Design review of the part built by this model. Coordinates are the model's own, in mm. Face numbers are marked on the shaded views. A direction names the side the tool comes from. Give positions to 0.01 mm unless a question says otherwise; leave off trailing zeros. Write each loop counter-clockwise with the first axis right and the second up, starting at its lowest first coordinate (ties: lowest second). Pieces come first, ordered by that corner, then holes. Notation, with made-up numbers: M 43,61 L 71,61 A15 cw 71,73 Z; hole C 81.25,68.25 d10. An arc over 180 degrees is marked long. One line per item, written item: value. Start each with the question number.
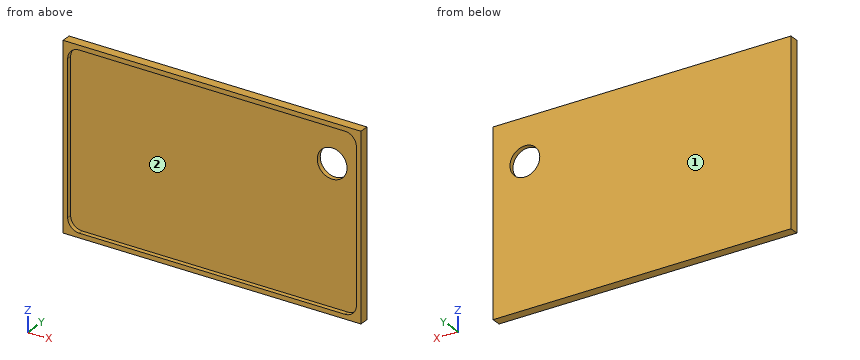
```python
from build123d import *

# Parameters (mm, degrees)
SKETCH1_W           = 65
SKETCH1_H           = 40
BOSS_EXTRUDE1_DEPTH = 45
SHELL1_T            = -1
SKETCH2_R           = 5
CUT_EXTRUDE1_DEPTH  = 8
SKETCH3_R           = 7.5
CUT_EXTRUDE2_DEPTH  = 8
FILLET1_R           = 2
FILLET2_R           = 2.5
SKETCH5_W           = 66.843722153
SKETCH5_H           = 46.578661822
CUT_EXTRUDE3_DEPTH  = 250
SKETCH7_W           = 65
SKETCH7_H           = 40
BOSS_EXTRUDE3_DEPTH = 1
SKETCH8_R           = 3.25
CUT_EXTRUDE4_DEPTH  = 7


with BuildPart() as part:
    # Sketch1 → Boss-Extrude1 (new body)
    with BuildSketch(Plane(origin=(0, 0, 0), x_dir=(1, 0, 0), z_dir=(0, 1, 0))):
        Rectangle(SKETCH1_W, SKETCH1_H)
    extrude(amount=BOSS_EXTRUDE1_DEPTH)

    # Shell1
    shell1_openings = [part.faces().sort_by_distance(p)[0] for p in [
        (0, 45, 0),
    ]]
    offset(amount=SHELL1_T, openings=shell1_openings, kind=Kind.INTERSECTION)

    # Sketch2 → Cut-Extrude1 (cut)
    with BuildSketch(Plane(origin=(32.5, 0, 0), x_dir=(0, 0, -1), z_dir=(1, 0, 0))):
        with Locations((0, 26)):
            Circle(SKETCH2_R)
    extrude(amount=-CUT_EXTRUDE1_DEPTH, mode=Mode.SUBTRACT)

    # Sketch3 → Cut-Extrude2 (cut)
    with BuildSketch(Plane.XZ):
        with Locations(Location((0, 0, 0), (0, 0, 270))):
            Circle(SKETCH3_R)
    extrude(amount=-CUT_EXTRUDE2_DEPTH, mode=Mode.SUBTRACT)

    # Fillet1
    # the kernel refuses this fillet: 2 mm, written as the material it adds along each edge
    with BuildSketch(Plane(origin=(31.5, 1, 19), x_dir=(0, 1, 0), z_dir=(0, 0, -1)), Plane(origin=(-31.5, 1, -19), x_dir=(0, 1, 0), z_dir=(0, 0, 1))) as fillet1_piece_1:
        with BuildLine():
            CenterArc((FILLET1_R, -FILLET1_R), FILLET1_R, 90, 90)
            Line((0, -FILLET1_R), (0, 0))
            Line((0, 0), (FILLET1_R, 0))
        make_face()
    extrude(amount=38)
    with BuildSketch(Plane(origin=(31.5, 1, -19), x_dir=(0, 1, 0), z_dir=(-1, 0, 0)), Plane(origin=(-31.5, 1, 19), x_dir=(0, 1, 0), z_dir=(1, 0, 0))) as fillet1_piece_2:
        with BuildLine():
            CenterArc((FILLET1_R, -FILLET1_R), FILLET1_R, 90, 90)
            Line((0, -FILLET1_R), (0, 0))
            Line((0, 0), (FILLET1_R, 0))
        make_face()
    extrude(amount=63)
    # the kernel refuses this fillet: 2 mm, written as the material it takes off along each edge
    with BuildSketch(Plane(origin=(0, 1, 0), x_dir=(0, 0, -1), z_dir=(-1, 0, 0))) as fillet1_2_piece_1:
        with BuildLine():
            CenterArc((9.232050808, 2), FILLET1_R, 210, 60)
            Line((9.232050808, 0), (7.5, 0))
            Line((7.5, 0), (7.5, 1))
        make_face()
    revolve(axis=Axis((0, 1, 0), (0, -1, 0)), mode=Mode.SUBTRACT)

    # Fillet2
    # the kernel refuses this fillet: 2.5 mm, written as the material it adds along each edge
    with BuildSketch(Plane(origin=(-29, 1, -16.5), x_dir=(-1, 0, 0), z_dir=(0, 0, 1))) as fillet2_piece_1:
        with BuildLine():
            CenterArc((0.5, -2), 2, 0, 90)
            Line((2.5, -2), (2.5, 0))
            Line((2.5, 0), (0.5, 0))
        make_face()
    revolve(axis=Axis((-29, 1, -16.5), (0, -1, 0)), revolution_arc=90)
    with BuildSketch(Plane(origin=(29, 1, -16.5), x_dir=(0, 0, -1), z_dir=(-1, 0, 0))) as fillet2_piece_2:
        with BuildLine():
            CenterArc((0.5, -2), 2, 0, 90)
            Line((2.5, -2), (2.5, 0))
            Line((2.5, 0), (0.5, 0))
        make_face()
    revolve(axis=Axis((29, 1, -16.5), (0, -1, 0)), revolution_arc=90)
    with BuildSketch(Plane(origin=(-29, 1, 16.5), x_dir=(0, 0, 1), z_dir=(1, 0, 0))) as fillet2_piece_3:
        with BuildLine():
            CenterArc((0.5, -2), 2, 0, 90)
            Line((2.5, -2), (2.5, 0))
            Line((2.5, 0), (0.5, 0))
        make_face()
    revolve(axis=Axis((-29, 1, 16.5), (0, -1, 0)), revolution_arc=90)
    with BuildSketch(Plane(origin=(29, 1, 16.5), x_dir=(1, 0, 0), z_dir=(0, 0, -1))) as fillet2_piece_4:
        with BuildLine():
            CenterArc((0.5, -2), 2, 0, 90)
            Line((2.5, -2), (2.5, 0))
            Line((2.5, 0), (0.5, 0))
        make_face()
    revolve(axis=Axis((29, 1, 16.5), (0, -1, 0)), revolution_arc=90)
    with BuildSketch(Plane(origin=(31.5, 1, 19), x_dir=(0, 0, -1), z_dir=(0, 1, 0)), Plane(origin=(31.5, 1, -19), x_dir=(-1, 0, 0), z_dir=(0, 1, 0)), Plane(origin=(-31.5, 45, 19), x_dir=(0, 0, -1), z_dir=(0, -1, 0))) as fillet2_piece_5:
        with BuildLine():
            CenterArc((FILLET2_R, FILLET2_R), FILLET2_R, 180, 90)
            Line((0, FILLET2_R), (0, 0))
            Line((0, 0), (FILLET2_R, 0))
        make_face()
    extrude(amount=44)
    with BuildSketch(Plane(origin=(-31.5, 1, -19), x_dir=(1, 0, 0), z_dir=(0, 1, 0))) as fillet2_piece_6:
        with BuildLine():
            CenterArc((FILLET2_R, -FILLET2_R), FILLET2_R, 90, 90)
            Line((0, -FILLET2_R), (0, 0))
            Line((0, 0), (FILLET2_R, 0))
        make_face()
    extrude(amount=44)

    # Sketch5 → Cut-Extrude3 (cut)
    with BuildSketch(Plane.XY.offset(20)):
        with Locations((0.921861077, 20.710669089)):
            Rectangle(SKETCH5_W, SKETCH5_H)
    extrude(amount=-CUT_EXTRUDE3_DEPTH, mode=Mode.SUBTRACT)

    # Sketch7 → Boss-Extrude3 (add)
    with BuildSketch(Plane(origin=(0, 45, 0), x_dir=(1, 0, 0), z_dir=(0, 1, 0))):
        Rectangle(SKETCH7_W, SKETCH7_H)
    extrude(amount=BOSS_EXTRUDE3_DEPTH)

    # Sketch8 → Cut-Extrude4 (cut)
    with BuildSketch(Plane(origin=(0, 46, 0), x_dir=(1, 0, 0), z_dir=(0, 1, 0))):
        with Locations(Location((25.564279631, -10.838515608, 0), (0, 0, 270))):
            Circle(SKETCH8_R)
    extrude(amount=-CUT_EXTRUDE4_DEPTH, mode=Mode.SUBTRACT)


solid = part.part
```
Q1. Take a section at D-D, the plane x = 23.5. Give the boundary of the cut face in (y, z), then the cut area to 3 significant figures.
Q2. Take a section at C-C, the plane z = 0.5. Give the boundary of the cut face in (x, y).
Q3. Take a section at B-B, the plane x = -7.5. Give the boundary of the cut face in (y, z), then the cut area to 3 significant figures.
Q4. Take a section at A-A, the plane y = 44.35. Give the boundary of the cut face in (x, z), then the cut area to 3 significant figures.
Q5. Machinability: for the marked faces 1 and 2, which of the approach directions +Z, -Z, +X, -X, +Y, -Y give a long, thin tool a straight path to every point of the face, cutting with its end or side? Answer none if there is none.
Q6. For P1, Ø2, axis at x = 10.5, z = 9.5, coming from the -Y side, flat-tipped, find the tip position at first contact; note if it passes through.
Q7. Wall thickness on line 1 (Z direction, x = 16, y = 44.35); line 2 (Y direction, x = -25.5, z = -9); line 3 (X direction, y = 44.7, z = -10): over which ranges is each line inside the solid? List them lowest first. Write a range as from..to.
Results list:
1. outline: M 44,-20 L 46,-20 L 46,8.33 L 45,8.33 L 45,-19 L 44,-19 Z; M 44,19 L 45,19 L 45,13.35 L 46,13.35 L 46,20 L 44,20 Z
1. area: 37.0 mm^2
2. outline: M -32.5,44 L -31.5,44 L -31.5,45 L 31.5,45 L 31.5,44 L 32.5,44 L 32.5,46 L -32.5,46 Z
3. outline: M 44,-20 L 46,-20 L 46,20 L 44,20 L 44,19 L 45,19 L 45,-19 L 44,-19 Z
3. area: 42.0 mm^2
4. outline: M -32.5,-20 L 32.5,-20 L 32.5,20 L -32.5,20 Z; hole M -31.5,-16.5 A2.5 ccw -29,-19 L 29,-19 A2.5 ccw 31.5,-16.5 L 31.5,16.5 A2.5 ccw 29,19 L -29,19 A2.5 ccw -31.5,16.5 Z
4. area: 211 mm^2
5. face 1: +Z, -Z, +X, -X, +Y
5. face 2: -Y
6. P1: stops at y = 45
7. line 1: z = -20..-19, 19..20
7. line 2: y = 45..46
7. line 3: x = -32.5..-31.5, 31.5..32.5
